Model file for the job. Use its own axes, mm. A direction names the side the tool comes from. Round coordinates to 2 decimals unless told otherwise and drop trailing zeros. Order: outer loops, then holes, each group sorted by start corner. A loop starts at its lowest first (then second) coordinate and runs counter-clockwise, first axis right, second up. Notation, with made-up numbers: (78.25, 48.25) -> (110.25, 48.25) arc R24 ccw to (110.25, 77.25) -> close; hole circle Ø5 at (36, 11). An arc over 180 degrees is marked (long way). Use CSV: the item, a comma, the result in double quotes.
Autodesk Inventor part; units mm, degrees
ref_plane "YZ Plane" through (0, 0, 0) normal (1, 0, 0) x (0, 1, 0)
ref_plane "XZ Plane" through (0, 0, 0) normal (0, 1, 0) x (-1, 0, 0)
ref_plane "XY Plane" through (0, 0, 0) normal (0, 0, 1) x (1, 0, 0)
sketch "Sketch1" plane through (0, 0, 0) normal (0, 1, 0) x (-1, 0, 0)
  circle A0 centre (0, 0) radius 12.5
  dimension "d0" = 25
extrude "Extrusion1" add sketch "Sketch1" along normal blind 49.5
hole "ReliefTop" at (0, 49.5, 0) direction (0, -1, 0) diameter 13.97 depth 0.254 countersink diameter 14.478 countersink angle 90
hole "ReliefBottom" at (0, 0, 0) direction (0, 1, 0) diameter 13.97 depth 0.254 countersink diameter 14.478 countersink angle 90
hole "MountBottomM6" at (0, 0.254, 0) direction (0, 1, 0) diameter 4.917 depth 7.366 tip angle 118 countersink diameter 5.508 countersink angle 90
hole "MountTopM4" at (0, 49.246, 0) direction (0, -1, 0) diameter 3.242 depth 14.478 tip angle 118 countersink diameter 3.808 countersink angle 90
sketch "Sketch2" plane through (0, 0, 0) normal (0, 0, 1) x (1, 0, 0)
  circle A0 centre (0, 20) radius 3
  line L0 (-12.5, 0) -> (12.5, 0)
  line L1 (0, -4.6) -> (0, 27.6)
  point P0 (0, 0)
  dimension "d49" = 6
  dimension "d50" = 20
extrude "Extrusion2" cut sketch "Sketch2" along normal through all both and the other way through all
chamfer "Chamfer1" distance 0.313 angle 45 2 edges at (-3, 19.9998, 12.1347) (-3, 19.9998, -12.1347)
equation "\"d1\" = height"
equation "\"d5\" = reliefMinor"
equation "\"d7\" = reliefMajor"
equation "\"d10\" = reliefDepth"
equation "\"d14\" = reliefMinor"
equation "\"d16\" = reliefMajor"
equation "\"d19\" = reliefDepth"
equation "\"d25\" = chamferM6"
equation "\"d28\" = depthM6"
equation "\"d40\" = chamferM4"
equation "\"d43\" = depthM4"
equation "\"reliefDepth\" = 0.254"
equation "\"reliefMinor\" = 13.97"
equation "\"reliefMajor\" = 14.478"
equation "\"chamferM6\" = 5.508"
equation "\"chamferM4\" = 3.808"
equation "\"depthM6\" = 7.366"
equation "\"depthM4\" = 14.478"
equation "\"height\" = 49.5"
properties part number "PLS-P642H0495A00_M" material "Stainless Steel"
Q1. Mould opens along Z. For faces 4 (the flat face through (-5.4, 0, -5.4)), 5 (the conical face through (0.13, 8.84, -0.41)), 6 (the cylindrical face through (-11.923, 24.404, -3.755)) say: +Z half, -Z half, draft (parallel to the pull), parting line (faces both ways), or undercut.
From the geometry:
face 4,"draft"
face 5,"undercut"
face 6,"parting line"
Q2. Which spindle directions (+Z, -Z, +X, -X, +Y, -Y) get a long thin tool onto all of the face, cutting with end or side? Do faces 1 (the flat face through (-5.4, 49.5, -5.4)), 2 (the cylindrical face through (-0.738, 4.134, -2.345)), 3 (the flat face through (1.5, 49.246, 1.5)). Say none if no direction does.
From the geometry:
face 1,"+Z, -Z, +X, -X, +Y"
face 2,"-Y"
face 3,"+Y"
Q3. Cut at A-A (z = 8.25). Give the cut face in (x, y).
From the geometry:
outline,"(-9.39, 0) -> (9.39, 0) -> (9.39, 49.5) -> (-9.39, 49.5) -> close; hole circle Ø6 at (0, 20)"
Q4. Cut at C-C (x = 9). Give the cut face in (y, z).
From the geometry:
outline,"(0, -8.67) -> (49.5, -8.67) -> (49.5, 8.67) -> (0, 8.67) -> close"
Q5. Cut at B-B (x = -10.5). Give the cut face in (y, z), plus the area to 3 significant figures.
From the geometry:
outline,"(0, -6.78) -> (49.5, -6.78) -> (49.5, 6.78) -> (0, 6.78) -> close"
area,"671 mm²"
Q6. Pin check, flat tips, straight feed: pin 1 (10 mm diameter, centred on x = 7.5, y = 23.5, fed in from +Z); pin 2 (12 mm diameter, centred on y = 43.5, z = 6.5, fed in from +X); pin 3 (1 mm diameter, centred on y = 10.5, z = 8.5, fed in from -X). Stop position of each tip, or through.
From the geometry:
pin 1,"stops at z = 12.25"
pin 2,"stops at x = 12.49"
pin 3,"stops at x = -9.6"
Q7. Probe line 1 along Y through (x, z) = (0, -3.25); line 2 along Z through (x, y) = (0, 38.75); line 3 along Y through (x, z) = (-2.5, -5). List the from-to ranges inside material, lowest first.
From the geometry:
line 1,"y = 0.25 to 17, 23 to 49.25"
line 2,"z = -12.5 to -1.62, 1.62 to 12.5"
line 3,"y = 0.25 to 18.34, 21.66 to 49.25"
